from build123d import *

# Parameters (mm, degrees)
F0_W        = 103.0951477587
F0_H        = 37.4727938324
F1_DEPTH    = 25.4
F2_R        = 9.8872931358
F3_DEPTH    = 165.1
F4_W        = 89.5363204181
F4_H        = 17.8772863001
F5_DEPTH    = 398.78
F6_T1_DEPTH = 464.6450864339
F7_SIZE2    = 116.84
F7_SIZE     = 15.24


# Not quite as in the source:
# - a fillet or chamfer that OpenCascade refuses, or shapes differently, is made with other operations: its cross-section is extruded or revolved along the edge and cut away or added


with BuildPart() as f1:
    # F0 (on Front) → F1 (new body)
    with BuildSketch(Plane.XZ):
        with Locations((-7.6333563775, 1.8935641274)):
            Rectangle(F0_W, F0_H)
    extrude(amount=F1_DEPTH)

    # F2 (on face) → F3 (join)
    with BuildSketch(Plane(origin=(0, 0, 0), x_dir=(-1, 0, 0), z_dir=(0, 1, 0))):
        Circle(F2_R)
    extrude(amount=F3_DEPTH)

    # F4 (on face) → F5 (join)
    with BuildSketch(Plane.XZ.offset(25.4)):
        with Locations((-8.1669483334, 2.3263469338)):
            Rectangle(F4_W, F4_H)
    extrude(amount=F5_DEPTH)

    # F6: chamfer of 25.4 x 10.16 on 4 edges, made by hand

    # F6_s2 → F6_t1 (cut)
    with BuildSketch(Plane.XZ.offset(25.4)):
        Polygon((-52.9351085424, 3.5477037838), (-27.5351085424, -6.6122962162), (-52.9351085424, -6.6122962162), align=None)
        Polygon((-27.5351085424, 11.2649900839), (-52.9351085424, 1.1049900839), (-52.9351085424, 11.2649900839), align=None)
        Polygon((11.2012118757, -6.6122962162), (36.6012118757, 3.5477037838), (36.6012118757, -6.6122962162), align=None)
        Polygon((11.2012118757, 11.2649900839), (36.6012118757, 1.1049900839), (36.6012118757, 11.2649900839), align=None)
    extrude(amount=F6_T1_DEPTH, mode=Mode.SUBTRACT)

    # F7 (call 1 of 2: OpenCascade refuses the feature's edges together)
    f7_edges = [f1.edges().sort_by_distance(p)[0] for p in [
        (-38.708412, -424.18, -2.142975),
        (-38.708412, -424.18, 6.795669),
    ]]
    f7_side = f1.faces().sort_by_distance((-8.166948, -424.18, 2.326347))[0]
    chamfer(f7_edges, length=F7_SIZE, length2=F7_SIZE2, reference=f7_side)

    # F7#2 (call 2 of 2)
    f7_2_edges = [f1.edges().sort_by_distance(p)[0] for p in [
        (22.374516, -424.18, -2.142975),
        (22.374516, -424.18, 6.795669),
    ]]
    f7_2_side = f1.faces().sort_by_distance((-8.166948, -424.18, 2.326347))[0]
    chamfer(f7_2_edges, length=F7_SIZE, length2=F7_SIZE2, reference=f7_2_side)


solid = f1.part
Could you check a few things on this model? Use its own coordinates, in mm. A direction names the side the tool comes from. Coordinates: 2 decimals unless noted, no trailing zeros. Order: outer loops, then holes, each group sorted by start corner. A loop starts at its lowest first (then second) coordinate and runs counter-clockwise, first axis right, second up. Notation, with made-up numbers: (79, -39.5) - (84, -39.5) arc R27 ccw to (84, -9.5) - close; hole circle Ø9 at (80, -16). An arc over 180 degrees is marked (long way). Answer in a Markdown table with one row per item. Add a question column.
(1) If we section it at B-B, the plane y = -43: Please give me the cut outline in (x, z) (3 decimals).
(2) On a 3-axis mill with a long thin cutter (end or side, diameter ignored), from which of +Z, -Z, +X, -X, +Y, -Y can I reach the whole of each face in a straight line? I mean faces 1 (the face through (-8, -25.4, 15)), 2 (the face through (22.218, -164.396, -2.206)), 3 (the face through (-38.55, -164.4, 6.86)), 4 (the face through (-38.865, -164.396, -2.08)). Say none if no direction works.
(3) If we section it at A-A, the plane x = 0: Please give me the cut outline in (y, z) (3 decimals), then the cut area to 3 significant figures.
(4) If we section it at D-D, the plane y = -336.5: Please give me the cut outline in (x, z) (3 decimals).
(5) I need wall thicknesses on L1, parallel to Y at x = 10, z = -13; L2, parallel to Z at x = 0, y = -81 (3 decimals); L3, parallel to Z at x = -21, y = -388. Which ranges of each line are inside material? Lowest first, please.
(6) Will these pins go through, and if not, where does the flat tip stop? pin 1 (3 mm diameter, centred on y = -215, z = 10.5, fed in from +X); pin 2 (3 mm diameter, centred on y = -218.5, z = 9.5, fed in from +X); pin 3 (6 mm diameter, centred on x = -19.5, z = -10, fed in from +Y).
(7) If we section it at C-C, the plane x = -39.5: Please give me the cut outline in (y, z).
Results are:
| question | item | result |
|---|---|---|
| 1 | outline | (-49.882, 2.326) - (-27.535, -6.612) - (11.201, -6.612) - (33.548, 2.326) - (11.201, 11.265) - (-27.535, 11.265) - close |
| 2 | face 1 | -Y |
| 2 | face 2 | -Z, +X, -Y |
| 2 | face 3 | +Z, -X, -Y |
| 2 | face 4 | -Z, -X, -Y |
| 3 | outline | (-402.862, 2.326) - (-339.234, -6.612) - (-25.4, -6.612) - (-25.4, -16.843) - (0, -16.843) - (0, -9.887) - (165.1, -9.887) - (165.1, 9.887) - (0, 9.887) - (0, 20.63) - (-25.4, 20.63) - (-25.4, 11.265) - (-339.234, 11.265) - close |
| 3 | area | 10,400 mm2 |
| 4 | outline | (-39.641, 2.326) - (-17.294, -6.612) - (0.96, -6.612) - (23.307, 2.326) - (0.96, 11.265) - (-17.294, 11.265) - close |
| 5 | L1 | y = -25.4 to 0 |
| 5 | L2 | z = -6.612 to 11.265 |
| 5 | L3 | z = 2.1 to 2.55 |
| 6 | pin 1 | stops at x = 16.86 |
| 6 | pin 2 | stops at x = 19.36 |
| 6 | pin 3 | stops at y = 0 |
| 7 | outline | (-336.9, 2.33) - (-307.34, -1.83) - (-25.4, -1.83) - (-25.4, -16.84) - (0, -16.84) - (0, 20.63) - (-25.4, 20.63) - (-25.4, 6.48) - (-307.34, 6.48) - close |
